from build123d import *

# Parameters (mm, degrees)
F0_W     = 25
F0_H     = 40
F1_DEPTH = 12.5


with BuildPart() as f1:
    # F0 (on Front) → F1 (new body, symmetric)
    with BuildSketch(Plane.XZ):
        with BuildLine():
            ThreePointArc((30.943819, 17.62255), (0.943819, 47.62255), (-29.056181, 17.62255))
            Line((-29.056181, 17.62255), (30.943819, 17.62255))
        make_face()
        Polygon((30.943819, 17.62255), (-29.056181, 17.62255), (-29.056181, -22.37745), (-11.556181, -22.37745), (13.443819, -22.37745), (30.943819, -22.37745), align=None)
        with Locations((0.943819, -42.37745)):
            Rectangle(F0_W, F0_H)
    extrude(amount=F1_DEPTH, both=True)


solid = f1.part
Input: part model. Units: mm. Frame: model coordinates. A direction names the side the tool comes from. Give positions to 0.01 mm unless a question says otherwise; leave off trailing zeros. Loops run counter-clockwise (first coordinate to the right, second up) from the corner with the lowest first, then second, coordinate; pieces in that order, holes last. Notation, with made-up numbers: M 80.5,0 L 91.5,0 A26 cw 91.5,38 Z; hole C 27,-7.75 d9. An arc over 180 degrees is marked long. Use one line per item in the form item = value.
1. First-contact query: pin 1 (4 mm diameter, centred on x = -5.5, y = -9.5, fed in from +Z); pin 2 (6 mm diameter, centred on x = 20.5, y = 6, fed in from -Z); pin 3 (2 mm diameter, centred on x = 11, y = 7.5, fed in from +Z). Flat tips, straight axial feed; report the tip coordinate or a pass-through.
Numbers:
pin_1 = 47.29
pin_2 = -22.38
pin_3 = 46.22
2. Reachability of faces 1 (the face through (1, 12.5, 6)), 2 (the face through (-20, 0, -22.377)), 3 (the face through (13.444, 0, -43)) from +Z, -Z, +X, -X, +Y, -Y: full face, straight path, thin tool, end or side. Return the list, or none.
Numbers:
face_1 = +Z, -Z, +X, -X, +Y
face_2 = -Z, -X, +Y, -Y
face_3 = -Z, +X, +Y, -Y
3. Section query C-C, the plane x = 26. Return the cut outline in (y, z).
Numbers:
outline = M -12.5,-22.38 L 12.5,-22.38 L 12.5,34.12 L -12.5,34.12 Z
4. Section query B-B, the plane x = -25. Return the cut outline in (y, z).
Numbers:
outline = M -12.5,-22.38 L 12.5,-22.38 L 12.5,32.69 L -12.5,32.69 Z
5. Line query: L1, parallel to X at y = -2.5, z = -37.5; L2, parallel to X at y = 6.75, z = 18.5; L3, parallel to Z at x = 9.5, y = -6. Output: solid intervals per line, ascending.
Numbers:
L1 = -11.56 to 13.44
L2 = -29.04 to 30.93
L3 = -62.38 to 46.38
6. Section query A-A, the plane y = -0.25. Return the cut outline in (x, z), and give its area (3 significant figures).
Numbers:
outline = M -29.06,-22.38 L -11.56,-22.38 L -11.56,-62.38 L 13.44,-62.38 L 13.44,-22.38 L 30.94,-22.38 L 30.94,17.62 A30 ccw -29.06,17.62 Z
area = 4,810 mm²
